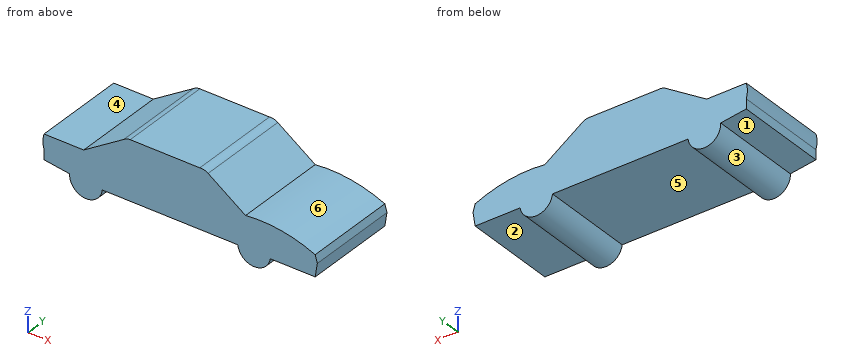
from build123d import *

# Parameters (mm, degrees)
F1_DEPTH = 33


with BuildPart() as f1:
    # F0 (on Front) → F1 (new body)
    with BuildSketch(Plane.XZ):
        with BuildLine():
            Line((0, 0), (53.250462, 0))
            Line((53.250462, 0), (26.834896, 18.175164))
            ThreePointArc((26.834896, 18.175164), (24.032478, 19.439506), (20.964772, 19.642696))
            Line((20.964772, 19.642696), (0, 19.642696))
            Line((0, 19.642696), (0, 0))
        make_face()
        with BuildLine():
            Line((40.881537, -12.428519), (53.250462, 0))
            Line((53.250462, 0), (0, 0))
            Line((0, 0), (0, -21.872539))
            Line((0, -21.872539), (37.131179, -21.872539))
            ThreePointArc((37.131179, -21.872539), (39.914753, -17.511266), (40.881537, -12.428519))
        make_face()
        with BuildLine():
            ThreePointArc((102.331229, -7.44311), (78.288954, -0.436962), (53.250462, 0))
            Line((53.250462, 0), (40.881537, -12.428519))
            ThreePointArc((40.881537, -12.428519), (39.914753, -17.511266), (37.131179, -21.872539))
            Line((37.131179, -21.872539), (47.805394, -21.872539))
            ThreePointArc((47.805394, -21.872539), (58.662919, -9.104587), (70.828642, -20.632885))
            ThreePointArc((70.828642, -20.632885), (70.793542, -21.532446), (70.688458, -22.426536))
            Line((70.688458, -22.426536), (102.331229, -22.426536))
            Line((102.331229, -22.426536), (103.862944, -12.71904))
            Line((103.862944, -12.71904), (102.331229, -7.44311))
        make_face()
        Polygon((0, -21.872539), (0, 0), (-34.451738, 0), (-30.538321, -21.872539), align=None)
        with BuildLine():
            Line((-34.451738, 0), (0, 0))
            Line((0, 0), (0, 19.642696))
            Line((0, 19.642696), (-28.115999, 19.642696))
            ThreePointArc((-28.115999, 19.642696), (-30.540046, 19.222817), (-32.681651, 18.012105))
            Line((-32.681651, 18.012105), (-60.890865, 0))
            Line((-60.890865, 0), (-34.451738, 0))
        make_face()
        with BuildLine():
            Line((-30.538321, -21.872539), (-34.451738, 0))
            Line((-34.451738, 0), (-60.890865, 0))
            Line((-60.890865, 0), (-88.844784, 0))
            ThreePointArc((-88.844784, 0), (-89.626398, -5.317535), (-88.844784, -10.63507))
            Line((-88.844784, -10.63507), (-88.844784, -17.421953))
            Line((-88.844784, -17.421953), (-70.805212, -19.897746))
            ThreePointArc((-70.805212, -19.897746), (-58.915888, -9.093747), (-47.738646, -20.632885))
            ThreePointArc((-47.738646, -20.632885), (-47.755345, -21.25361), (-47.805394, -21.872539))
            Line((-47.805394, -21.872539), (-30.538321, -21.872539))
        make_face()
        with BuildLine():
            ThreePointArc((70.828642, -20.632885), (58.662919, -9.104587), (47.805394, -21.872539))
            ThreePointArc((47.805394, -21.872539), (59.004222, -32.174501), (70.688458, -22.426536))
            ThreePointArc((70.688458, -22.426536), (70.793542, -21.532446), (70.828642, -20.632885))
        make_face()
        with BuildLine():
            ThreePointArc((-70.805212, -19.897746), (-60.271278, -32.135561), (-47.805394, -21.872539))
            ThreePointArc((-47.805394, -21.872539), (-47.755345, -21.25361), (-47.738646, -20.632885))
            ThreePointArc((-47.738646, -20.632885), (-58.915888, -9.093747), (-70.805212, -19.897746))
        make_face()
    extrude(amount=F1_DEPTH)

    # F2: F1 across plane


with BuildPart() as f1_1:
    add(f1.part)
    add(f1.part.mirror(Plane.XZ))


solid = f1_1.part
The model under review builds one solid part; all positions refer to its coordinate system, in mm. Face numbers are marked on the shaded views. A direction names the side the tool comes from. Round coordinates to 2 decimals unless told otherwise and drop trailing zeros. Order: outer loops, then holes, each group sorted by start corner. A loop starts at its lowest first (then second) coordinate and runs counter-clockwise, first axis right, second up. Notation, with made-up numbers: (62, 81) -> (91, 81) arc R28 ccw to (91, 117) -> close; hole circle Ø11 at (88.5, 59). An arc over 180 degrees is marked (long way). Use CSV: the item, a comma, the result in double quotes. Start each with the question number.
(1) Consider section C-C on x = 9. Write out the cut boundary in (y, z).
(2) Consider section D-D on z = -2.5. Write out the cut boundary in (x, y).
(3) Mouldability with a two-part tool opening along X and no side actions: class the marked faces 1, 2 and 3 as pulls with the +X half, pulls with the -X half, needs draft (parallel to the pull), parting line crosses it, or undercut.
(4) Consider section B-B on y = 19. Write out the cut boundary in (x, z) (3 decimals), and give its area (3 significant figures).
(5) Tool access review of the marked faces 4, 5 and 6: name each direction out of +Z, -Z, +X, -X, +Y, -Y from which nothing blocks a thin tool from reaching the whole face with its end or side.
(6) Wall thickness on probe 1 along Z at (x, y) = (-13.5, -13); probe 2 along X at (y, z) = (-3, -26); probe 3 along Z at (x, y) = (54.5, -9): over which ranges is each line inside the solid? List them lowest first. Write a range as from..to.
(7) Insertion check: pin 1 (2 mm diameter, centred on y = -19.5, z = -24, fed in from -X); pin 2 (1 mm diameter, centred on x = -66.5, y = -23, fed in from +Z); pin 3 (3 mm diameter, centred on x = 82, y = -17.5, fed in from -Z); pin 4 (12 mm diameter, centred on x = -2.5, z = -22.5, fed in from +Y). Each pin has a flat end and moves straight along its axis. Give the tip position at first contact, or say it passes through.
(8) Consider section A-A on z = -26. Write out the cut boundary in (x, y).
Responses:
1,outline,"(-33, -21.87) -> (33, -21.87) -> (33, 19.64) -> (-33, 19.64) -> close"
2,outline,"(-89.41, -33) -> (88.24, -33) -> (88.24, 33) -> (-89.41, 33) -> close"
3,face 1,"pulls with the -X half"
3,face 2,"needs draft"
3,face 3,"undercut"
4,outline,"(-88.845, -17.422) -> (-70.805, -19.898) arc R11.545 ccw to (-47.805, -21.873) -> (47.805, -21.873) arc R11.545 ccw to (70.688, -22.427) -> (102.331, -22.427) -> (103.863, -12.719) -> (102.331, -7.443) arc R94.384 ccw to (53.25, 0) -> (26.835, 18.175) arc R8.641 ccw to (20.965, 19.643) -> (-28.116, 19.643) arc R7.207 ccw to (-32.682, 18.012) -> (-60.891, 0) -> (-88.845, 0) arc R18.479 ccw to (-88.845, -10.635) -> close"
4,area,"6,110 mm²"
5,face 4,"+Z, -X, +Y, -Y"
5,face 5,"-Z, +Y, -Y"
5,face 6,"+Z, +Y, -Y"
6,probe 1,"-21.87..19.64"
6,probe 2,"-69.51..-49.06, 49.06..69.51"
6,probe 3,"-31.14..0.14"
7,pin 1,"x = -70.58"
7,pin 2,"z = 0"
7,pin 3,"z = -22.43"
7,pin 4,"y = 33"
8,outline,"(-69.51, -33) -> (-49.06, -33) -> (-49.06, 33) -> (-69.51, 33) -> close; (49.06, -33) -> (69.51, -33) -> (69.51, 33) -> (49.06, 33) -> close"
